Job drawing, mm, ordinate dimensions from the low corner. One solid piece. Coordinates: 2 decimals unless noted, no trailing zeros. Order: outer loops, then holes, each group sorted by start corner. A loop starts at its lowest first (then second) coordinate and runs counter-clockwise, first axis right, second up. Notation, with made-up numbers: (-26, -31.75) - (-6, -31.75) arc R23 cw to (-6, 1.25) - close; hole circle Ø5 at (38, 73). An arc over 180 degrees is marked (long way). Use a Markdown table: item, result. Add a question column.
1) Drop flat-ended pins along their axis: P1, Ø12, axis at x = 43.5, z = 109, coming from the -Y side; P2, Ø2, axis at x = 123, y = 138.5, coming from the +Z side. Give the stop position or say it passes through.
2) Saw through at B-B on x = 124. List the corners of the cut face in (y, z) (1 decimal), then the cut area to 3 significant figures.
3) Saw through at D-D on y = 162. List the corners of the cut face in (x, z).
4) Saw through at C-C on x = 175.5. List the corners of the cut face in (y, z).
5) Saw through at A-A on y = 103. List the corners of the cut face in (x, z).
6) Wall check: L1, parallel to Z at x = 31.5, y = 96.5. Give the ranges that are in metal, low to high. Write a range as [from, to].
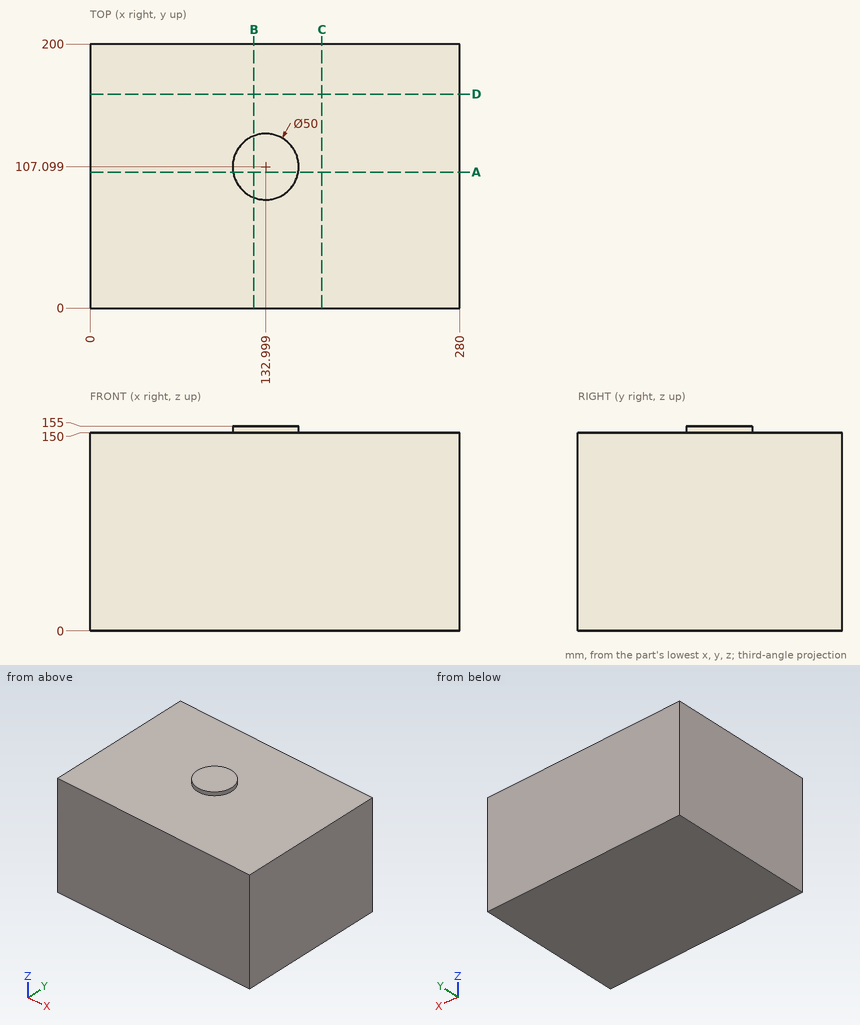
Results are:
| question | item | result |
|---|---|---|
| 1 | P1 | y = 0 |
| 1 | P2 | z = 150 |
| 2 | outline | (0, 0) - (200, 0) - (200, 150) - (130.4, 150) - (130.4, 155) - (83.8, 155) - (83.8, 150) - (0, 150) - close |
| 2 | area | 30,200 mm2 |
| 3 | outline | (0, 0) - (280, 0) - (280, 150) - (0, 150) - close |
| 4 | outline | (0, 0) - (200, 0) - (200, 150) - (0, 150) - close |
| 5 | outline | (0, 0) - (280, 0) - (280, 150) - (157.66, 150) - (157.66, 155) - (108.34, 155) - (108.34, 150) - (0, 150) - close |
| 6 | L1 | [0, 150] |
